Read the model definition and answer for the solid it produces. Units are mm, in the model's axes. A direction names the side the tool comes from. Round coordinates to 2 decimals unless told otherwise and drop trailing zeros. Order: outer loops, then holes, each group sorted by start corner. A loop starts at its lowest first (then second) coordinate and runs counter-clockwise, first axis right, second up. Notation, with made-up numbers: (-14.5, 47.25) - (-9.5, 47.25) arc R28 ccw to (-9.5, 86.25) - close; hole circle Ø2 at (-6.75, 78). An arc over 180 degrees is marked (long way). One line per question, with ' | ' between items. Start each with the question number.
1) The mould has two halves that part along Z. Classify faces 1 (the flat face through (-137.12, -2, 2)), 2 (the flat face through (-0.595, -2, -56)), 3 (the flat face through (-126, -2, -72.418)), 4 (the flat face through (17, -2, -31.143)): pulls with the +Z half, pulls with the -Z half, needs draft (parallel to the pull), parting line crosses it, or undercut.
2) The part is cut by section A-A, the plane z = -53. Give the vertices of the cut face in (x, y) (3 decimals).
3) Flat-ended cylindrical pins translate along their axes: pin 1 (1 mm diameter, centred on x = -99.5, y = -1.5, fed in from -Z); pin 2 (1.6 mm diameter, centred on y = -2.5, z = -71, fed in from +X); pin 3 (1 mm diameter, centred on x = 17, y = -1, fed in from +Z). Find the tip coordinate at first contact, or state that the pin passes through.
4) The part is cut by section C-C, the plane x = -107.5. Give the vertices of the cut face in (y, z) (3 decimals).
5) The part is cut by section D-D, the plane z = 2.5. Give the vertices of the cut face in (x, y) (3 decimals).
6) The part is cut by section B-B, the plane x = -37. Give the vertices of the cut face in (y, z) (3 decimals).
7) Straight lines are drawn through the part: line 1 (Z direction, x = -36, y = -2.85); line 2 (Z direction, x = -34, y = -0.95); line 3 (Z direction, x = -60, y = -1.15). For each, find the intervals that lie inside material, in ascending order. Write a range as from..to.
8) For faces 5 (the flat face through (-20, -2, -49.805)), 6 (the flat face through (17, -2, -5.743)), 7 (the flat face through (-86.32, -2, 9)), 8 (the flat face through (17, -2, -43.843)), 9 (the flat face through (-139, -2, -5.743)), determine the directions among +Z, -Z, +X, -X, +Y, -Y from which every point of the face is accessible in a straight line to the end or side of a thin tool.
from build123d import *

# Parameters (mm, degrees)
F1_DEPTH = 3.175
F2_W     = 38.1
F2_H     = 12.7
F3_DEPTH = 25.4


# Not quite as in the source:
# - a length typed as a fraction of an inch, garbled in the dataset ("3 / 203.2 mm" for 3/8 in), is restored


with BuildPart() as f1:
    # F0 (on Front) → F1 (new body)
    with BuildSketch(Plane.XZ):
        Polygon((15.2796131081, -5.7429333596), (15.2796131081, 6.9570666404), (-10.1203868919, 6.9570666404), (-10.1203868919, 10.1320666404), (-35.5203868919, 10.1320666404), (-35.5203868919, 6.9570666404), (-60.9203868919, 6.9570666404), (-60.9203868919, 10.1320666404), (-86.3203868919, 10.1320666404), (-86.3203868919, 6.9570666404), (-111.7203868919, 6.9570666404), (-111.7203868919, 10.1320666404), (-137.1203868919, 10.1320666404), (-137.1203868919, 6.9570666404), (-137.1203868919, -5.7429333596), (-140.2953868919, -5.7429333596), (-140.2953868919, -18.4429333596), (-137.1203868919, -18.4429333596), (-137.1203868919, -31.1429333596), (-140.2953868919, -31.1429333596), (-140.2953868919, -43.8429333596), (-137.1203868919, -43.8429333596), (-137.1203868919, -56.5429333596), (-140.2953868919, -56.5429333596), (-140.2953868919, -69.2429333596), (-140.2953868919, -72.4179333596), (-137.1203868919, -72.4179333596), (-111.7203868919, -72.4179333596), (-111.7203868919, -69.2429333596), (-86.3203868919, -69.2429333596), (-86.3203868919, -72.4179333596), (-60.9203868919, -72.4179333596), (-60.9203868919, -69.2429333596), (-35.5203868919, -69.2429333596), (-35.5203868919, -72.4179333596), (-10.1203868919, -72.4179333596), (-10.1203868919, -69.2429333596), (15.2796131081, -69.2429333596), (18.4546131081, -69.2429333596), (18.4546131081, -56.5429333596), (15.2796131081, -56.5429333596), (15.2796131081, -43.8429333596), (18.4546131081, -43.8429333596), (18.4546131081, -31.1429333596), (15.2796131081, -31.1429333596), (15.2796131081, -18.4429333596), (18.4546131081, -18.4429333596), (18.4546131081, -5.7429333596), align=None)
    extrude(amount=F1_DEPTH)

    # F2 (on face) → F3 (cut)
    with BuildSketch(Plane.XZ.offset(3.175)):
        with Locations((-19.6453868919, -56.1550986022)):
            Rectangle(F2_W, F2_H)
    extrude(amount=-F3_DEPTH, mode=Mode.SUBTRACT)


solid = f1.part
Values:
1) face 1: needs draft | face 2: undercut | face 3: pulls with the -Z half | face 4: undercut
2) outline: (-137.12, -3.175) - (-38.695, -3.175) - (-38.695, 0) - (-137.12, 0) - close; (-0.595, -3.175) - (15.28, -3.175) - (15.28, 0) - (-0.595, 0) - close
3) pin 1: stops at z = -69.24 | pin 2: stops at x = -10.12 | pin 3: stops at z = -5.74
4) outline: (-3.175, -69.243) - (0, -69.243) - (0, 6.957) - (-3.175, 6.957) - close
5) outline: (-137.12, -3.175) - (15.28, -3.175) - (15.28, 0) - (-137.12, 0) - close
6) outline: (-3.175, -69.243) - (0, -69.243) - (0, -62.505) - (-3.175, -62.505) - close; (-3.175, -49.805) - (0, -49.805) - (0, 6.957) - (-3.175, 6.957) - close
7) line 1: z = -69.24..-62.51, -49.81..6.96 | line 2: z = -72.42..-62.51, -49.81..10.13 | line 3: z = -69.24..6.96
8) face 5: +Y, -Y | face 6: +Z, +X, +Y, -Y | face 7: +Z, +Y, -Y | face 8: +X, +Y, -Y | face 9: +Z, -X, +Y, -Y
